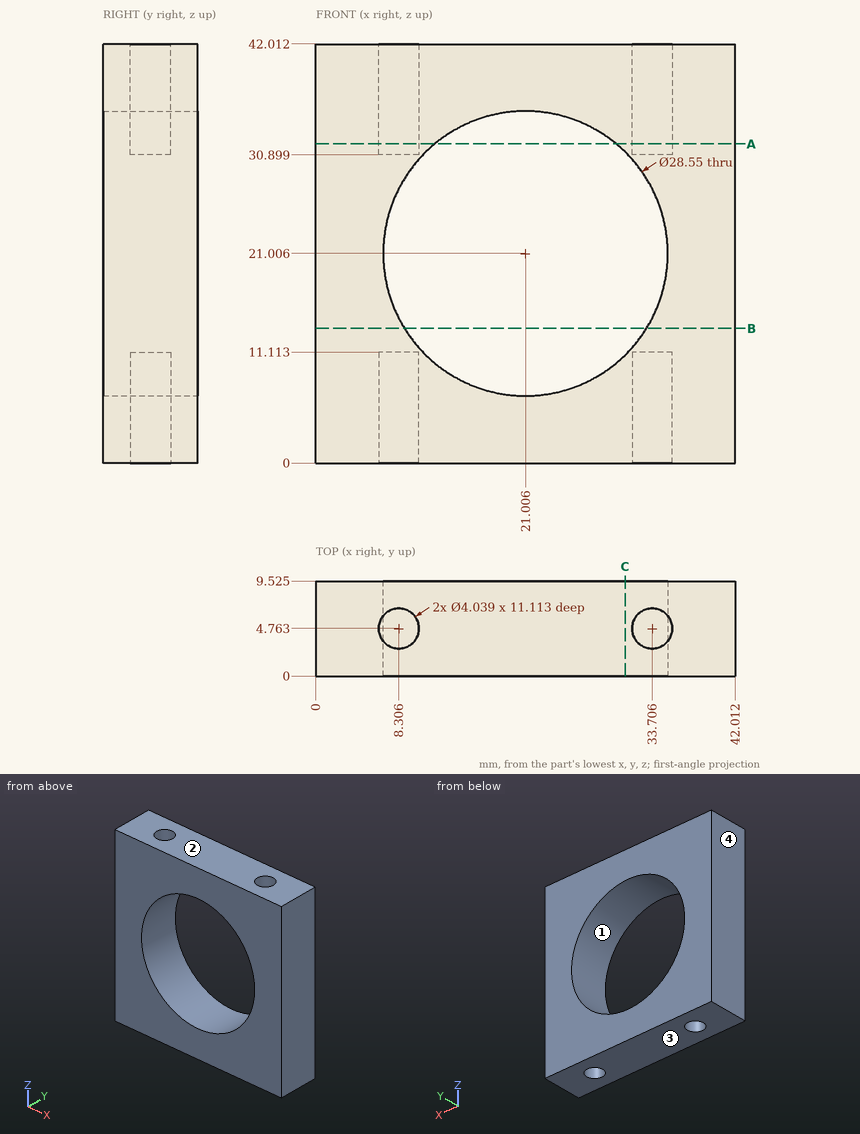
Answer from the drawing. Dimensions are ordinates in mm from the lowest x, y and z of the part. Give positions to 0.01 mm unless a question says otherwise; leave off trailing zeros. Write each loop counter-clockwise with the first axis right and the second up, starting at its lowest first coordinate (ties: lowest second). Pieces come first, ordered by that corner, then holes. Notation, with made-up numbers: (5.25, 51) - (18.25, 51) arc R19 cw to (18.25, 74) - close; hole circle Ø4 at (82, 23). An arc over 180 degrees is marked (long way). One line per item, written item: value. Start each with the question number.
1. Find section B-B (z = 13.5). Write down the section's boundary in (x, y) (1 decimal), then the cut area to 3 significant figures.
2. For a pull along Z with two mould halves and no side action, classify the marked faces 1, 2, 3 and 4 as +Z half, -Z half, draft (parallel to the pull), parting line (faces both ways), or undercut.
3. Consider probe 1 along X at (y, z) = (6.5, 36) (1 decimal); probe 2 along X at (y, z) = (6.25, 11) (1 decimal); probe 3 along Z at (x, y) = (11, 3.25) (1 decimal). Determine where each line is inside the solid, lowest interval first.
4. Find section A-A (z = 32). Write down the section's boundary in (x, y) (1 decimal).
5. Given pin 1 (3.5 mm diameter, centred on x = 8.31, y = 4.76, fed in from +Z); pin 2 (2.5 mm diameter, centred on x = 8.31, y = 4.76, fed in from -Z), each flat-ended and moving along its own axis, determine where each tip first touches the part or whether it passes through.
6. Find section C-C (x = 31). Write down the section's boundary in (y, z) (1 decimal).
Geometry results:
1. outline: (0, 0) - (8.9, 0) - (8.9, 9.5) - (0, 9.5) - close; (33.1, 0) - (42, 0) - (42, 9.5) - (33.1, 9.5) - close
1. area: 169 mm2
2. face 1: undercut
2. face 2: +Z half
2. face 3: -Z half
2. face 4: draft
3. probe 1: 0 to 7.3, 9.3 to 32.7, 34.7 to 42
3. probe 2: 0 to 6.9, 9.7 to 10.8, 31.2 to 32.3, 35.1 to 42
3. probe 3: 0 to 10.8, 31.2 to 42
4. outline: (0, 0) - (11.9, 0) - (11.9, 9.5) - (0, 9.5) - close; (30.1, 0) - (42, 0) - (42, 9.5) - (30.1, 9.5) - close; hole circle Ø4 at (8.3, 4.8); hole circle Ø4 at (33.7, 4.8)
5. pin 1: z = 30.9
5. pin 2: z = 11.11
6. outline: (0, 0) - (9.5, 0) - (9.5, 10.8) - (0, 10.8) - close; (0, 31.2) - (9.5, 31.2) - (9.5, 42) - (0, 42) - close
